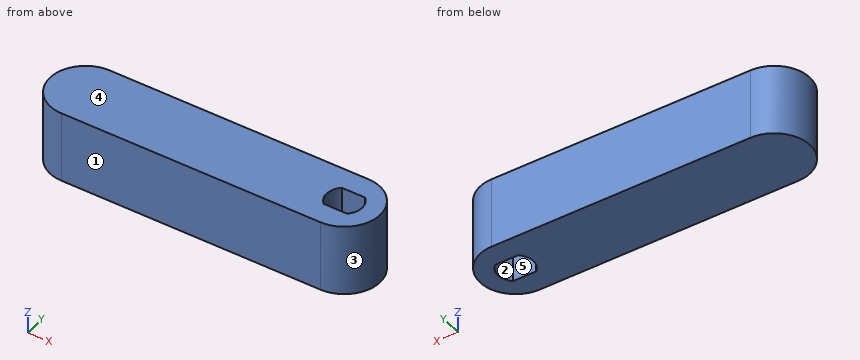
from build123d import *

# Parameters (mm, degrees)
SKETCH1_R           = 8
SKETCH1_R_2         = 4
BOSS_EXTRUDE1_DEPTH = 16


with BuildPart() as part:
    # Sketch1 → Boss-Extrude1 (new body)
    # profile 1 of 5: a face of its own
    with BuildSketch(Plane.XY):
        with Locations((-59, 0)):
            Circle(SKETCH1_R)
    # profile 2 of 5: a face of its own
    with BuildSketch(Plane.XY):
        with BuildLine():
            ThreePointArc((0, -8), (-8, 0), (0, 8))
            Line((0, 8), (-59, 8))
            ThreePointArc((-59, 8), (-53.343145751, 5.656854249), (-51, 0))
            ThreePointArc((-51, 0), (-53.343145751, -5.656854249), (-59, -8))
            Line((-59, -8), (0, -8))
        make_face()
    # profile 3 of 5: a face of its own
    with BuildSketch(Plane.XY):
        Circle(SKETCH1_R)
        Circle(SKETCH1_R_2, mode=Mode.SUBTRACT)
    # profile 4 of 5: a face of its own
    with BuildSketch(Plane.XY):
        with BuildLine():
            Line((-2.645751311, 3), (2.645751311, 3))
            ThreePointArc((2.645751311, 3), (0, 4), (-2.645751311, 3))
        make_face()
    # profile 5 of 5: a face of its own
    with BuildSketch(Plane.XY):
        with BuildLine():
            ThreePointArc((-2.645751311, -3), (0, -4), (2.645751311, -3))
            Line((2.645751311, -3), (-2.645751311, -3))
        make_face()
    extrude(amount=-BOSS_EXTRUDE1_DEPTH)


solid = part.part
Read the model definition and answer for the solid it produces. Units are mm, in the model's axes. Face numbers are marked on the shaded views. A direction names the side the tool comes from. Give positions to 0.01 mm unless a question says otherwise; leave off trailing zeros. Write each loop counter-clockwise with the first axis right and the second up, starting at its lowest first coordinate (ties: lowest second). Pieces come first, ordered by that corner, then holes. Notation, with made-up numbers: (-8.5, 6) - (3.5, 6) arc R10 cw to (3.5, 14) - close; hole circle Ø6 at (-30.5, 41.25). An arc over 180 degrees is marked (long way). Use CSV: the item, a comma, the result in double quotes. Start each with the question number.
(1) Find section A-A (y = 0). Give the vertices of the cut face in (x, z), plus the area to 3 significant figures.
(2) Consider line 1 along Y through (x, z) = (-0.5, -13); line 2 along X through (y, z) = (0, -2); line 3 along Y through (x, z) = (2.5, -4.75). Determine where each line is inside the solid, lowest interval first.
(3) Determine the mould class of the marked faces 1, 2 and 3 for opening direction Y: +Y half, -Y half, draft (parallel to the pull), parting line (faces both ways), or undercut.
(4) Find section B-B (z = -1.25). Give the vertices of the cut face in (x, y).
(5) For the marked faces 4 and 5, determine the directions among +Z, -Z, +X, -X, +Y, -Y from which every point of the face is accessible in a straight line to the end or side of a thin tool.
(6) Given P1, Ø2, axis at y = -4, z = -4.5, coming from the -X side; P2, Ø8, axis at y = -6.5, z = -3, coming from the +X side, each flat-ended and moving along its own axis, determine where each tip first touches the part or whether it passes through.
(7) Find section D-D (y = -6). Give the vertices of the cut face in (x, z), plus the area to 3 significant figures.
(8) Find section C-C (y = 5). Give the vertices of the cut face in (x, z) (3 decimals), plus the area to 3 significant figures.
Findings below:
1,outline,"(-67, -16) - (-4, -16) - (-4, 0) - (-67, 0) - close; (4, -16) - (8, -16) - (8, 0) - (4, 0) - close"
1,area,"1,070 mm2"
2,line 1,"-8 to -3, 3 to 8"
2,line 2,"-67 to -4, 4 to 8"
2,line 3,"-7.6 to -3, 3 to 7.6"
3,face 1,"-Y half"
3,face 2,"undercut"
3,face 3,"parting line"
4,outline,"(-59, -8) - (0, -8) arc R8 ccw to (0, 8) - (-59, 8) arc R8 ccw to start; hole (-2.65, -3) - (2.65, -3) arc R4 ccw to (2.65, 3) - (-2.65, 3) arc R4 ccw to start"
5,face 4,"+Z, +X, -X, +Y, -Y"
5,face 5,"+Z, -Z"
6,P1,"x = -66.42"
6,P2,"x = 7.6"
7,outline,"(-64.29, -16) - (5.29, -16) - (5.29, 0) - (-64.29, 0) - close"
7,area,"1,110 mm2"
8,outline,"(-65.245, -16) - (6.245, -16) - (6.245, 0) - (-65.245, 0) - close"
8,area,"1,140 mm2"
